Geometry check sheet. Reference: the model listing, model coordinates, mm. A direction names the side the tool comes from. Give positions to 0.01 mm unless a question says otherwise; leave off trailing zeros. Write each loop counter-clockwise with the first axis right and the second up, starting at its lowest first coordinate (ties: lowest second). Pieces come first, ordered by that corner, then holes. Notation, with made-up numbers: M 82,-36.75 L 118,-36.75 A20 ccw 118,-20.75 Z; hole C 19.5,-22 d11. An arc over 180 degrees is marked long. One line per item, written item: value. Start each with the question number.
1. Tool access check on faces 1 (the face through (0, 13, -10)), 2 (the face through (29, 10.3, -17.6)), 3 (the face through (4.737, 4.738, -11.341)). Record the directions out of +Z, -Z, +X, -X, +Y, -Y that give a thin tool (end or side, any length) a straight path to the whole face; none if there is none.
2. Scan lines: line 1 (Y direction, x = 6.35, z = -12.75); line 2 (X direction, y = 15, z = -12); line 3 (Z direction, x = 5.5, y = 9.75). Record each from-to range of solid material in increasing order.
3. Cross-section at C-C on x = 6.35. Record the cut outline in (y, z), then the cut area to 3 significant figures.
4. Cross-section at B-B on y = 5. Count the separate pieces of the cut face and the enclosed holes in it, then the cut area to 3 significant figures.
5. Release check for a two-part mould opening along Y. For faces 4 (the face through (14.8, 1.72, -16.6)), 5 (the face through (15.056, 12.677, -17.449)), 6 (the face through (26.4, 4.78, -32.92)) record: pulls with the +Y half, pulls with the -Y half, needs draft (parallel to the pull), parting line crosses it, or undercut.
6. Gauge pin test, flat ends, axial feed: pin 1 (5 mm diameter, centred on x = 29, z = -27, fed in from -Y); pin 2 (5 mm diameter, centred on x = 31.5, z = -16, fed in from +Y); pin 3 (5 mm diameter, centred on y = 4, z = -12, fed in from +X); pin 4 (5.5 mm diameter, centred on x = 6.35, y = 5.97, fed in from -Z). Record the tip position at first contact, or that the pin passes through.
from build123d import *

# Parameters (mm, degrees)
SKETCH2_W               = 12.7
SKETCH2_H               = 22.225
SKETCH2_R               = 2.032
BOSS_EXTRUDE1_DEPTH     = 12.7
BOSS_EXTRUDE2_DEPTH     = 22.225
CUT_EXTRUDE1_DEPTH      = 55.959756427
CUT_EXTRUDE1_DEPTH_BACK = 55.959756427
SKETCH5_R               = 2.286
CUT_EXTRUDE2_DEPTH      = 55.959756427
CUT_EXTRUDE2_DEPTH_BACK = 55.959756427
FILLET1_START           = -2.63267612
FILLET1_DEPTH           = 17.0815
FILLET1_START_2         = 1.720391704
FILLET1_2_DEPTH         = 23.279608296
FILLET1_3_DEPTH         = 22.225
FILLET1_START_3         = -3.948943888
FILLET1_4_DEPTH         = 21.90945623


with BuildPart() as part:
    # Sketch2 → Boss-Extrude1 (new body)
    with BuildSketch(Plane.XY):
        with Locations((6.35, 12.832891704)):
            Rectangle(SKETCH2_W, SKETCH2_H)
        with Locations((6.35, 15.499891704)):
            Circle(SKETCH2_R, mode=Mode.SUBTRACT)
        with Locations((6.35, 5.974891704)):
            Circle(SKETCH2_R, mode=Mode.SUBTRACT)
    extrude(amount=BOSS_EXTRUDE1_DEPTH)

    # Sketch4 → Boss-Extrude2 (add)
    with BuildSketch(Plane(origin=(0, 23.945391704, 0), x_dir=(1, 0, 0), z_dir=(0, 1, 0))):
        Polygon((28.798929105, -28.031967319), (13.083480893, -12.316519107), (20.941204999, -4.458795001), (36.656653211, -20.174243213), (38.632309558, -18.198586866), (22.916861346, -2.483138654), (25.4, 0), (12.7, 0), (12.7, -12.7), (0, -12.7), (10.838416863, -14.561583137), (26.553865075, -30.277031349), align=None)
    extrude(amount=-BOSS_EXTRUDE2_DEPTH)

    # Sketch5 → Cut-Extrude1 (cut, two sides: drawn at the far end of the back side and taken through both)
    with BuildSketch(Plane(origin=(-1.861583137, 0, 1.861583137), x_dir=(0.7071067811865527, 0, 0.7071067811865424), z_dir=(-0.7071067811865424, 0, 0.7071067811865527)).offset(-CUT_EXTRUDE1_DEPTH_BACK)):
        with Locations((36.243802071, 5.657391696)):
            Circle(SKETCH5_R)
    extrude(amount=CUT_EXTRUDE1_DEPTH + CUT_EXTRUDE1_DEPTH_BACK, mode=Mode.SUBTRACT)

    # Sketch6 → Cut-Extrude2 (cut, two sides: drawn at the far end of the back side and taken through both)
    with BuildSketch(Plane(origin=(-1.861583137, 0, 1.861583137), x_dir=(0.7071067811865527, 0, 0.7071067811865424), z_dir=(-0.7071067811865424, 0, 0.7071067811865527)).offset(-CUT_EXTRUDE2_DEPTH_BACK)):
        with BuildLine():
            Line((17.960512242, 23.945391704), (40.185512242, 23.945391704))
            Line((40.185512242, 23.945391704), (40.185512242, 10.842113828))
            ThreePointArc((40.185512242, 10.842113828), (30.860575382, 20.425710965), (17.960512242, 23.945391704))
        make_face()
    extrude(amount=CUT_EXTRUDE2_DEPTH + CUT_EXTRUDE2_DEPTH_BACK, mode=Mode.SUBTRACT)

    # Fillet1: read off the stored shape, not the designer's step
    # Fillet1 outline → Fillet1 (cut)
    with BuildSketch(Plane(origin=(0, 0, 0), x_dir=(0.707106781186553, 0, 0.707106781186542), z_dir=(0.707106781186542, 0, -0.707106781186553)).offset(FILLET1_START)):
        with BuildLine():
            Line((40.185512242, -10.842113828), (40.185512242, -9.543914332))
            ThreePointArc((40.185512242, -9.543914332), (39.998674237, -10.864794174), (39.452819934, -12.082034938))
            ThreePointArc((39.452819934, -12.082034938), (39.827956058, -11.467268539), (40.185512242, -10.842113828))
        make_face()
    extrude(amount=FILLET1_DEPTH, mode=Mode.SUBTRACT)

    # Fillet1 2 outline → Fillet1 2 (cut)
    with BuildSketch(Plane(origin=(0, 0, 0), x_dir=(1, 0, 0), z_dir=(0, 1, 0)).offset(FILLET1_START_2)):
        with BuildLine():
            ThreePointArc((2.63753897, -13.153018013), (0.747340245, -12.070077877), (0, -10.023839104))
            Line((0, -10.023839104), (0, -12.7))
            Line((0, -12.7), (2.63753897, -13.153018013))
        make_face()
    extrude(amount=FILLET1_2_DEPTH, mode=Mode.SUBTRACT)

    # Fillet1 3 outline → Fillet1 3 (add)
    with BuildSketch(Plane(origin=(0, 0, 0), x_dir=(1, 0, 0), z_dir=(0, 1, 0)).offset(FILLET1_START_2)):
        with BuildLine():
            Line((10.838416863, -14.561583137), (2.884336106, -13.195407357))
            ThreePointArc((2.884336106, -13.195407357), (10.263075725, -15.672812319), (16.545160109, -20.268326383))
            Line((16.545160109, -20.268326383), (10.838416863, -14.561583137))
        make_face()
        with BuildLine():
            Line((22.916861346, -2.483138654), (26.166236401, -5.732513709))
            ThreePointArc((26.166236401, -5.732513709), (24.81331492, -2.995885603), (25.4, 0))
            Line((25.4, 0), (22.916861346, -2.483138654))
        make_face()
        with BuildLine():
            Line((20.941204999, -4.458795001), (17.573608954, -7.826391046))
            ThreePointArc((17.573608954, -7.826391046), (20.941205, -6.431487092), (24.308801045, -7.826391046))
            Line((24.308801045, -7.826391046), (20.941204999, -4.458795001))
        make_face()
        with BuildLine():
            ThreePointArc((16.451076939, -15.684115152), (15.056172984, -12.316519106), (16.451076939, -8.948923061))
            Line((16.451076939, -8.948923061), (13.083480893, -12.316519107))
            Line((13.083480893, -12.316519107), (16.451076939, -15.684115152))
        make_face()
    extrude(amount=FILLET1_3_DEPTH)

    # Fillet1 4 outline → Fillet1 4 (cut)
    with BuildSketch(Plane(origin=(0, 0, 0), x_dir=(0.707106781186553, 0, 0.707106781186542), z_dir=(0.707106781186542, 0, -0.707106781186553)).offset(FILLET1_START_3)):
        with BuildLine():
            Line((17.960512242, -23.945391704), (26.031065938, -23.945391704))
            Line((26.031065938, -23.945391704), (26.031065938, -22.629124036))
            ThreePointArc((26.031065938, -22.629124036), (22.049106057, -23.61416512), (17.960512242, -23.945391704))
        make_face()
    extrude(amount=FILLET1_4_DEPTH, mode=Mode.SUBTRACT)


with BuildPart() as body_2:
    # Mirror3: mirrored copy
    add(part.part.mirror(Plane(origin=(0, 0, -2.54), x_dir=(1, 0, 0), z_dir=(0, 0, -1))))


solid = body_2.part
Report:
1. face 1: +Z, -Z, -X, +Y, -Y
1. face 2: +Y, -Y
1. face 3: +Z
2. line 1: y = 1.72 to 3.94, 8.01 to 13.47, 17.53 to 23.95
2. line 2: x = 0 to 4.38, 8.32 to 18.84, 23.04 to 27.35
2. line 3: z = -18.87 to -5.08
3. outline: M 1.72,-19.12 L 23.95,-19.12 L 23.95,-5.08 L 17.53,-5.08 L 17.53,-17.78 L 13.47,-17.78 L 13.47,-5.08 L 8.01,-5.08 L 8.01,-17.78 L 3.94,-17.78 L 3.94,-5.08 L 1.72,-5.08 Z
3. area: 209 mm^2
4. separate pieces: 3
4. enclosed holes: 0
4. area: 334 mm^2
5. face 4: pulls with the -Y half
5. face 5: needs draft
5. face 6: undercut
6. pin 1: passes through
6. pin 2: stops at y = 22.09
6. pin 3: stops at x = 29.85
6. pin 4: stops at z = -20.19
